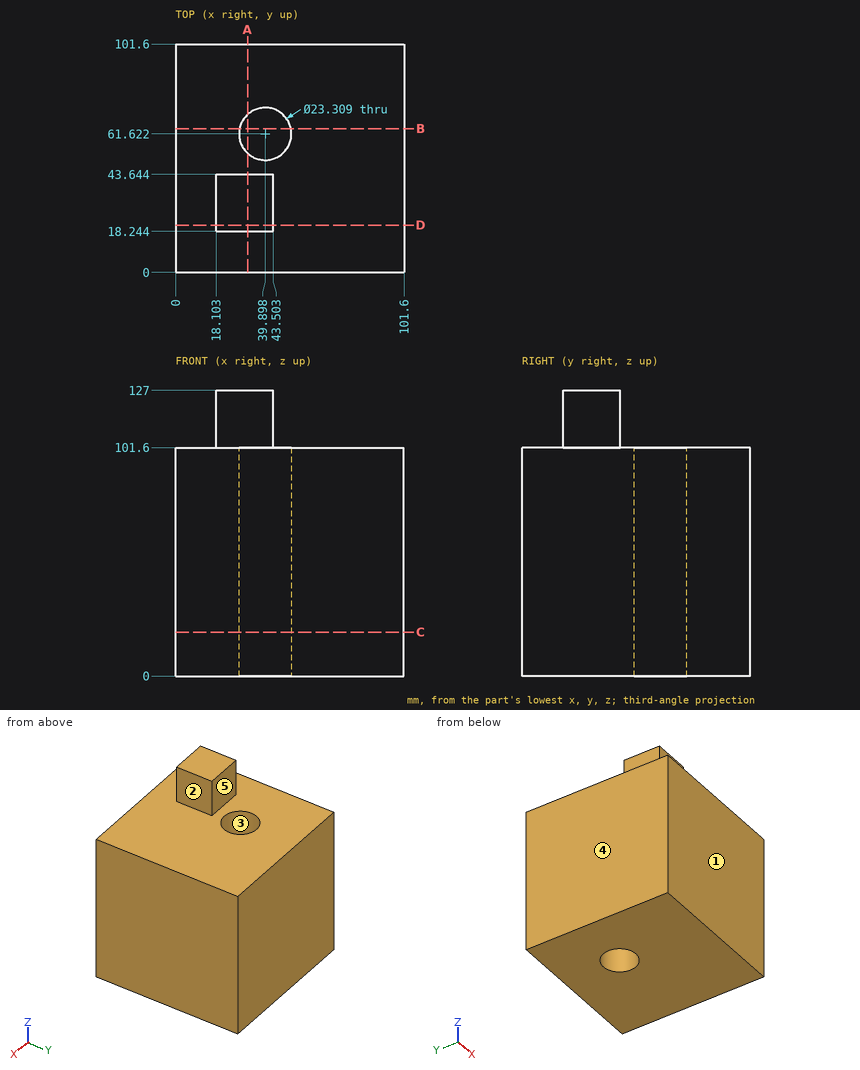
Study the drawing (mm; zero at the part's minimum x, y, z) and answer. A direction names the side the tool comes from. Coordinates: 2 decimals unless noted, no trailing zeros. Write each loop counter-clockwise with the first axis right and the second up, starting at its lowest first coordinate (ties: lowest second). Pieces come first, ordered by that corner, then holes.
Q1. Section B-B, the plane y = 64 is taken. Write down the section's boundary in (x, z), then the cut area to 3 significant figures.
Returned:
outline: (0, 0) - (28.49, 0) - (28.49, 101.6) - (0, 101.6) - close; (51.31, 0) - (101.6, 0) - (101.6, 101.6) - (51.31, 101.6) - close
area: 8,000 mm2
Q2. Section D-D, the plane y = 21 is taken. Write down the section's boundary in (x, z), then the cut area to 3 significant figures.
Returned:
outline: (0, 0) - (101.6, 0) - (101.6, 101.6) - (43.5, 101.6) - (43.5, 127) - (18.1, 127) - (18.1, 101.6) - (0, 101.6) - close
area: 11,000 mm2
Q3. Find the intervals of material crossed by line 1 along Z through (x, y) = (85.5, 56); line 2 along X through (y, z) = (71, 7.5) (1 decimal); line 3 along Y through (x, z) = (31.5, 10.5) (1 decimal), in increasing order.
Returned:
line 1: z = 0 to 101.6
line 2: x = 0 to 33, 46.8 to 101.6
line 3: y = 0 to 53.5, 69.7 to 101.6
Q4. Given P1, Ø2, axis at x = 75.5, y = 61.5, coming from the +Z side; P2, Ø20.5, axis at x = 30.5, z = 108, coming from the -Y side; P3, Ø7.5, axis at y = 29, z = 108, coming from the -X side, each flat-ended and moving along its own axis, determine where each tip first touches the part or whether it passes through.
Returned:
P1: stops at z = 101.6
P2: stops at y = 0
P3: stops at x = 18.1
Q5. The mould has two halves that part along Y. Classify the marked faces 1, 2 and 3: released by +Y, released by -Y, zero draft, split by the parting line, or undercut.
Returned:
face 1: released by -Y
face 2: zero draft
face 3: undercut
Q6. Section C-C, the plane z = 19.5 is taken. Write down the section's boundary in (x, y) (1 decimal).
Returned:
outline: (0, 0) - (101.6, 0) - (101.6, 101.6) - (0, 101.6) - close; hole circle Ø23.3 at (39.9, 61.6)
Q7. Section A-A, the plane x = 32 is taken. Write down the section's boundary in (y, z), then the cut area to 3 significant figures.
Returned:
outline: (0, 0) - (53.05, 0) - (53.05, 101.6) - (43.64, 101.6) - (43.64, 127) - (18.24, 127) - (18.24, 101.6) - (0, 101.6) - close; (70.19, 0) - (101.6, 0) - (101.6, 101.6) - (70.19, 101.6) - close
area: 9,230 mm2
Q8. Which of the six approach directions +Z, -Z, +X, -X, +Y, -Y give full straight-line access (tool end or side, diameter ignored) to the marked faces 4 and 5?
Returned:
face 4: +Z, -Z, -X, +Y, -Y
face 5: +Z, +X, -X, +Y
